Read the model definition and answer for the solid it produces. Units are mm, in the model's axes. A direction names the side the tool comes from. Coordinates: 2 decimals unless noted, no trailing zeros. Write each loop counter-clockwise with the first axis right and the second up, starting at its lowest first coordinate (ties: lowest second). Pieces come first, ordered by that corner, then holes.
(1) Which of the six approach directions +Z, -Z, +X, -X, +Y, -Y give full straight-line access (tool end or side, diameter ignored) to faces 1 (the cylindrical face through (-1.65, -7.44, 37.92)), 2 (the flat face through (0, 0, 0))?
(2) Section A-A on x = 0 is taken. Write down the section's boundary in (y, z).
(3) Find the intervals of material crossed by probe 1 along X at (y, z) = (5.5, 5); probe 2 along X at (y, z) = (-4, 45.5); probe 3 along Y at (x, z) = (0, 3), in increasing order.
(4) Section D-D on z = 30 is taken. Write down the section's boundary in (x, y).
(5) Section C-C on z = 18.5 is taken. Write down the section's boundary in (x, y).
(6) Given pin 1 (10 mm diameter, centred on x = -9.5, y = -9, fed in from -Z); pin 2 (5 mm diameter, centred on y = -5, z = 21, fed in from +X); pin 3 (2 mm diameter, centred on y = -4.5, z = 17.5, fed in from +X); pin 4 (2 mm diameter, centred on x = -9, z = 35.5, fed in from -Y), each flat-ended and moving along its own axis, determine where each tip first touches the part or whether it passes through.
from build123d import *

# Parameters (mm, degrees)
F0_R      = 12.7
F1_DEPTH  = 25.4
F2_R      = 5.08
F1_FACE_R = 7.62
F3_DEPTH  = 25.4


with BuildPart() as f1:
    # F0 (on Top) → F1 (new body)
    with BuildSketch(Plane.XY):
        Circle(F0_R)
    extrude(amount=F1_DEPTH)

    # F2
    f2_edges = [f1.edges().sort_by_distance(p)[0] for p in [
        (-12.7, 0, 25.4),
        (-12.7, 0, 0),
    ]]
    fillet(f2_edges, radius=F2_R)

    # F1_face (on face) → F3 (join)
    with BuildSketch(Plane.XY.offset(25.4)):
        Circle(F1_FACE_R)
    extrude(amount=F3_DEPTH)


solid = f1.part
Response:
1. face 1: +Z
1. face 2: -Z, +X, -X, +Y, -Y
2. outline: (-12.7, 5.08) arc R5.08 ccw to (-7.62, 0) - (7.62, 0) arc R5.08 ccw to (12.7, 5.08) - (12.7, 20.32) arc R5.08 ccw to (7.62, 25.4) - (7.62, 50.8) - (-7.62, 50.8) - (-7.62, 25.4) arc R5.08 ccw to (-12.7, 20.32) - close
3. probe 1: x = -11.45 to 11.45
3. probe 2: x = -6.49 to 6.49
3. probe 3: y = -12.25 to 12.25
4. outline: circle Ø15.24 at (0, 0)
5. outline: circle Ø25.4 at (0, 0)
6. pin 1: stops at z = 0.02
6. pin 2: stops at x = 12.44
6. pin 3: stops at x = 12.21
6. pin 4: passes through
